Could you check a few things on this model? Use its own coordinates, in mm. A direction names the side the tool comes from. Round coordinates to 2 decimals unless told otherwise and drop trailing zeros. Loops run counter-clockwise (first coordinate to the right, second up) from the corner with the lowest first, then second, coordinate; pieces in that order, holes last. Notation, with made-up numbers: (-33.5, 27) - (-29.5, 27) arc R19 ccw to (-29.5, 58) - close; hole circle Ø1 at (21, -11). An arc over 180 degrees is marked (long way). Answer as CSV lines item,"result". Start each with the question number.
1) Suppose I cut it at D-D, the plane y = -172.5. Write out the boundary of the cut face in (x, z).
2) Suppose I cut it at B-B, the plane z = -3.75. Write out the boundary of the cut face in (x, y).
3) Please list where these lines run through material, in increasing order: line 1 along X through (y, z) = (-166.5, -3.25); line 2 along Z through (x, y) = (-7, -132); line 3 along X through (y, z) = (-189.5, -7).
4) Suppose I cut it at C-C, the plane x = -1. Write out the boundary of the cut face in (y, z), then the cut area to 3 significant figures.
5) I'm going to push flat-ended pins straight in: pin 1 Ø4 at (x, y) = (2.5, -60.5) entering from -Z; pin 2 Ø0.5 at (y, z) = (-125, -0.5) entering from -X; pin 3 Ø4.5 at (x, y) = (-17.5, -131) entering from +Z; pin 4 Ø10 at (x, y) = (0, -66.5) entering from -Z. Where does each tip first touch, or does it pass through?
6) Suppose I cut it at A-A, the plane y = -124.5. Write out the boundary of the cut face in (x, z).
7) We'd pull the mould along Y, two halves only. Please class faces 5 (the face through (-0.3, -19.215, -0.7)), 6 (the face through (0.976, -162.787, -0.493)), 7 (the face through (18, -110, -6.5)): pulls with the +Y half, pulls with the -Y half, needs draft (parallel to the pull), parting line crosses it, or undercut.
8) Which directions (+Z, -Z, +X, -X, +Y, -Y) give clear straight access to the entire face, cutting with the end or side of a thin tool? Please do faces 1 (the face through (13.555, -108, -4)), 2 (the face through (18, -110, -7.5)), 3 (the face through (0.976, -102.787, -0.493)), 4 (the face through (14.555, -108, -4)).
```python
from build123d import *

# Parameters (mm, degrees)
SKETCH_2_W                         = 27
SKETCH_2_H                         = 180
SM_BASE_FLANGE_1_DEPTH             = 1
SM_EDGE_FLANGE_1_STRIP_W           = 5.4732
SM_EDGE_FLANGE_1_STRIP_H           = 1
SM_EDGE_FLANGE_1_STRIP_CUT_DEPTH   = 180
SM_EDGE_FLANGE_1_STRIP_2_W         = 5.4732
SM_EDGE_FLANGE_1_STRIP_2_H         = 1
SM_EDGE_FLANGE_1_STRIP_CUT_2_DEPTH = 180
SM_EDGE_FLANGE_1_DEPTH             = 180
SM_EDGE_FLANGE_1_BEND_DEPTH        = 180
SM_EDGE_FLANGE_2_STRIP_W           = 5.4732
SM_EDGE_FLANGE_2_STRIP_H           = 1
SM_EDGE_FLANGE_2_STRIP_CUT_DEPTH   = 180
SM_EDGE_FLANGE_2_STRIP_2_W         = 5.4732
SM_EDGE_FLANGE_2_STRIP_2_H         = 1
SM_EDGE_FLANGE_2_STRIP_CUT_2_DEPTH = 180
SM_EDGE_FLANGE_2_DEPTH             = 180
SM_EDGE_FLANGE_2_BEND_DEPTH        = 180
CUT_EXTRUDE_3_DEPTH                = 10
PATTERN_LINEAR_1_COUNT             = 9
PATTERN_LINEAR_1_PITCH             = 30


# Sheet-metal steps are written as plain solids
with BuildPart() as part:
    # 草图2 → 基体-法兰1 (new body)
    with BuildSketch(Plane.XY):
        with Locations((1.054557063, -109.215322961)):
            Rectangle(SKETCH_2_W, SKETCH_2_H)
    extrude(amount=-SM_BASE_FLANGE_1_DEPTH)

    # 边线-法兰1 strip (across the edge) → 边线-法兰1 strip cut (cut)
    with BuildSketch(Plane(origin=(-12.445442937, -199.215322961, -1), x_dir=(1, 0, 0), z_dir=(0, 1, 0))):
        with Locations((-1, -0.5)):
            Rectangle(SM_EDGE_FLANGE_1_STRIP_W, SM_EDGE_FLANGE_1_STRIP_H)
    extrude(amount=SM_EDGE_FLANGE_1_STRIP_CUT_DEPTH, mode=Mode.SUBTRACT)

    # 边线-法兰1 strip 2 (across the edge) → 边线-法兰1 strip cut 2 (cut)
    with BuildSketch(Plane(origin=(14.554557063, -19.215322961, -1), x_dir=(-1, 0, 0), z_dir=(0, -1, 0))):
        with Locations((-1, -0.5)):
            Rectangle(SM_EDGE_FLANGE_1_STRIP_2_W, SM_EDGE_FLANGE_1_STRIP_2_H)
    extrude(amount=SM_EDGE_FLANGE_1_STRIP_CUT_2_DEPTH, mode=Mode.SUBTRACT)

    # 边线-法兰1 section (across the edge) → 边线-法兰1 (add)
    with BuildSketch(Plane(origin=(-12.445442937, -199.215322961, -1), x_dir=(1, 0, 0), z_dir=(0, 1, 0))):
        with BuildLine():
            Line((0, 0.7366), (0, 6.5))
            Line((0, 6.5), (1, 6.5))
            Line((1, 6.5), (1, 0.7366))
            ThreePointArc((1, 0.7366), (1.215745145, 0.215745145), (1.7366, 0))
            Line((1.7366, 0), (1.7366, -1))
            ThreePointArc((1.7366, -1), (0.508638364, -0.491361636), (0, 0.7366))
        make_face()
    extrude(amount=SM_EDGE_FLANGE_1_DEPTH)

    # 边线-法兰1 section 2 (across the edge) → 边线-法兰1 bend (add)
    with BuildSketch(Plane(origin=(14.554557063, -19.215322961, -1), x_dir=(-1, 0, 0), z_dir=(0, -1, 0))):
        with BuildLine():
            Line((0, 0.7366), (0, 6.5))
            Line((0, 6.5), (1, 6.5))
            Line((1, 6.5), (1, 0.7366))
            ThreePointArc((1, 0.7366), (1.215745145, 0.215745145), (1.7366, 0))
            Line((1.7366, 0), (1.7366, -1))
            ThreePointArc((1.7366, -1), (0.508638364, -0.491361636), (0, 0.7366))
        make_face()
    extrude(amount=SM_EDGE_FLANGE_1_BEND_DEPTH)

    # 边线-法兰2 strip (across the edge) → 边线-法兰2 strip cut (cut)
    with BuildSketch(Plane(origin=(-12.445442937, -19.215322961, -7.5), x_dir=(0, 0, 1), z_dir=(0, -1, 0))):
        with Locations((-1, -0.5)):
            Rectangle(SM_EDGE_FLANGE_2_STRIP_W, SM_EDGE_FLANGE_2_STRIP_H)
    extrude(amount=SM_EDGE_FLANGE_2_STRIP_CUT_DEPTH, mode=Mode.SUBTRACT)

    # 边线-法兰2 strip 2 (across the edge) → 边线-法兰2 strip cut 2 (cut)
    with BuildSketch(Plane(origin=(14.554557063, -199.215322961, -7.5), x_dir=(0, 0, 1), z_dir=(0, 1, 0))):
        with Locations((-1, -0.5)):
            Rectangle(SM_EDGE_FLANGE_2_STRIP_2_W, SM_EDGE_FLANGE_2_STRIP_2_H)
    extrude(amount=SM_EDGE_FLANGE_2_STRIP_CUT_2_DEPTH, mode=Mode.SUBTRACT)

    # 边线-法兰2 section (across the edge) → 边线-法兰2 (add)
    with BuildSketch(Plane(origin=(-12.445442937, -19.215322961, -7.5), x_dir=(0, 0, 1), z_dir=(0, -1, 0))):
        with BuildLine():
            Line((0, 0.7366), (0, 6.5))
            Line((0, 6.5), (1, 6.5))
            Line((1, 6.5), (1, 0.7366))
            ThreePointArc((1, 0.7366), (1.215745145, 0.215745145), (1.7366, 0))
            Line((1.7366, 0), (1.7366, -1))
            ThreePointArc((1.7366, -1), (0.508638364, -0.491361636), (0, 0.7366))
        make_face()
    extrude(amount=SM_EDGE_FLANGE_2_DEPTH)

    # 边线-法兰2 section 2 (across the edge) → 边线-法兰2 bend (add)
    with BuildSketch(Plane(origin=(14.554557063, -199.215322961, -7.5), x_dir=(0, 0, 1), z_dir=(0, 1, 0))):
        with BuildLine():
            Line((0, 0.7366), (0, 6.5))
            Line((0, 6.5), (1, 6.5))
            Line((1, 6.5), (1, 0.7366))
            ThreePointArc((1, 0.7366), (1.215745145, 0.215745145), (1.7366, 0))
            Line((1.7366, 0), (1.7366, -1))
            ThreePointArc((1.7366, -1), (0.508638364, -0.491361636), (0, 0.7366))
        make_face()
    extrude(amount=SM_EDGE_FLANGE_2_BEND_DEPTH)

    # 草图17 → 切除-拉伸3 (cut)
    with BuildSketch(Plane.XY):
        with BuildLine():
            Line((4.626807443, -189.215322961), (4.626807443, -179.215322961))
            ThreePointArc((4.626807443, -179.215322961), (1.054557063, -175.643072581), (-2.517693316, -179.215322961))
            Line((-2.517693316, -179.215322961), (-2.517693316, -189.215322961))
            ThreePointArc((-2.517693316, -189.215322961), (1.054557063, -192.78757334), (4.626807443, -189.215322961))
        make_face()
    cut_extrude_3 = extrude(amount=-CUT_EXTRUDE_3_DEPTH, mode=Mode.SUBTRACT)

    # 阵列(线性)1: 切除-拉伸3 ×9
    with Locations(*[(0, i * PATTERN_LINEAR_1_PITCH, 0) for i in range(1, PATTERN_LINEAR_1_COUNT)]):
        add(cut_extrude_3, mode=Mode.SUBTRACT)


solid = part.part
```
Filled sheet:
1,outline,"(-18.95, -7.5) - (-13.18, -7.5) arc R1.74 ccw to (-11.45, -5.76) - (-11.45, -1.74) arc R0.74 cw to (-10.71, -1) - (12.82, -1) arc R0.74 cw to (13.55, -1.74) - (13.55, -5.76) arc R1.74 ccw to (15.29, -7.5) - (21.05, -7.5) - (21.05, -6.5) - (15.29, -6.5) arc R0.74 cw to (14.55, -5.76) - (14.55, -1.74) arc R1.74 ccw to (12.82, 0) - (-10.71, 0) arc R1.74 ccw to (-12.45, -1.74) - (-12.45, -5.76) arc R0.74 cw to (-13.18, -6.5) - (-18.95, -6.5) - close"
2,outline,"(-12.45, -199.22) - (-11.45, -199.22) - (-11.45, -19.22) - (-12.45, -19.22) - close; (13.55, -199.22) - (14.55, -199.22) - (14.55, -19.22) - (13.55, -19.22) - close"
3,line 1,"-12.45 to -11.45, 13.55 to 14.55"
3,line 2,"-1 to 0"
3,line 3,"-18.95 to -11.96, 14.07 to 21.05"
4,outline,"(-199.22, -1) - (-192.14, -1) - (-192.14, 0) - (-199.22, 0) - close; (-176.29, -1) - (-162.14, -1) - (-162.14, 0) - (-176.29, 0) - close; (-146.29, -1) - (-132.14, -1) - (-132.14, 0) - (-146.29, 0) - close; (-116.29, -1) - (-102.14, -1) - (-102.14, 0) - (-116.29, 0) - close; (-86.29, -1) - (-72.14, -1) - (-72.14, 0) - (-86.29, 0) - close; (-56.29, -1) - (-42.14, -1) - (-42.14, 0) - (-56.29, 0) - close; (-26.29, -1) - (-19.22, -1) - (-19.22, 0) - (-26.29, 0) - close"
4,area,"84.9 mm²"
5,pin 1,"through"
5,pin 2,"x = -12.14"
5,pin 3,"z = -6.5"
5,pin 4,"z = -1"
6,outline,"(-18.95, -7.5) - (-13.18, -7.5) arc R1.74 ccw to (-11.45, -5.76) - (-11.45, -1.74) arc R0.74 cw to (-10.71, -1) - (-2.52, -1) - (-2.52, 0) - (-10.71, 0) arc R1.74 ccw to (-12.45, -1.74) - (-12.45, -5.76) arc R0.74 cw to (-13.18, -6.5) - (-18.95, -6.5) - close; (4.63, -1) - (12.82, -1) arc R0.74 cw to (13.55, -1.74) - (13.55, -5.76) arc R1.74 ccw to (15.29, -7.5) - (21.05, -7.5) - (21.05, -6.5) - (15.29, -6.5) arc R0.74 cw to (14.55, -5.76) - (14.55, -1.74) arc R1.74 ccw to (12.82, 0) - (4.63, 0) - close"
7,face 5,"pulls with the +Y half"
7,face 6,"undercut"
7,face 7,"needs draft"
8,face 1,"-Z, +Y, -Y"
8,face 2,"-Z, +X, -X, +Y, -Y"
8,face 3,"+Z, -Z"
8,face 4,"+Z, +X, +Y, -Y"
